The listing builds one solid part. Answer for the finished solid, in the listing's coordinates (mm). Face numbers are marked on the shaded views. A direction names the side the tool comes from. Round coordinates to 2 decimals unless told otherwise and drop trailing zeros. Order: outer loops, then holes, each group sorted by start corner. A loop starts at its lowest first (then second) coordinate and runs counter-clockwise, first axis right, second up. Notation, with made-up numbers: (59, -26.5) -> (107, -26.5) arc R28 ccw to (107, 2.5) -> close; hole circle Ø4 at (-32.5, -14). An arc over 180 degrees is marked (long way). Return JSON: item names as keys, results as strings. Group by question number.
(1) The part is cut by section C-C (z = -7.5). Determine the outline of the cut face in (x, y).
(2) Consider line 1 (Y direction, x = 4.3, z = 0); line 2 (X direction, y = 3.75, z = -0.5); line 3 (X direction, y = 10.25, z = 0.75) (3 decimals). Determine where each line is inside the solid, lowest interval first. Write a range as [from, to].
(3) Each of these flat-tipped pins is pushed along its axis until it touches: pin 1 (0.7 mm diameter, centred on x = 4.5, z = 0, fed in from +Y); pin 2 (1.2 mm diameter, centred on x = 4.5, y = 3.5, fed in from -Z); pin 3 (0.8 mm diameter, centred on y = 10.5, z = 3.5, fed in from +X). Where does it stop, or does it pass through?
(4) Which of the six approach directions +Z, -Z, +X, -X, +Y, -Y give full straight-line access (tool end or side, diameter ignored) to the marked faces 1, 2 and 3?
(5) The part is cut by section B-B (x = 0). Determine the outline of the cut face in (y, z), plus the area to 3 significant figures.
(6) The part is cut by section A-A (z = 0). Determine the outline of the cut face in (x, y) (3 decimals), plus the area to 3 significant figures.
(7) The part is cut by section D-D (y = 5). Determine the outline of the cut face in (x, z), plus the area to 3 significant figures.
(8) Determine the mould class of the marked faces 4, 5 and 6 for opening direction Z: +Z half, -Z half, draft (parallel to the pull), parting line (faces both ways), or undercut.
from build123d import *

# Parameters (mm, degrees)
BOSS_EXTRUDE1_DEPTH       = 2.3
BOSS_EXTRUDE2_START       = 1
BOSS_EXTRUDE2_DEPTH       = 1
SKETCH19_W                = 2
SKETCH19_H                = 1.95
SKETCH19_R                = 0.45
SKETCH19_W_2              = 1.95
SKETCH19_H_2              = 2
CMOS_MOUNTING_HOLES_DEPTH = 3.3
FILLET1_R                 = 0.5
SKETCH21_W                = 7.2
SKETCH21_H                = 7.2
SKETCH21_W_2              = 6
SKETCH21_H_2              = 6
COLUMN_DEPTH              = 6.52
SKETCH22_W                = 6
SKETCH22_H                = 6
COLUMN_EXTRUDED_CUT_DEPTH = 14.675174588
COLUMN_OUTSIDE_FILLET_R   = 1.5
COLUMN_INSIDE_FILLET_R    = 1
SKETCH25_W                = 2.5
SKETCH25_H                = 2.5
SET_SCREW_EXTRUSION_DEPTH = 1.5
SET_SCREW_HOLE_REACH      = 21.834
SKETCH26_R                = 0.55
LARGE_START               = -3.3
SKETCH29_R                = 0.875
LARGE_WIRE_HOLE_DEPTH     = 3.3
FILLET3_R                 = 0.5


with BuildPart() as part:
    # Sketch4 → Boss-Extrude1 (new body)
    with BuildSketch(Plane(origin=(0, 9.37, 0), x_dir=(1, 0, 0), z_dir=(0, 1, 0))):
        with BuildLine():
            Line((-6.55, 5.65), (-6.55, -5.65))
            ThreePointArc((-6.55, -5.65), (-6.286396103, -6.286396103), (-5.65, -6.55))
            Line((-5.65, -6.55), (5.65, -6.55))
            ThreePointArc((5.65, -6.55), (6.286396103, -6.286396103), (6.55, -5.65))
            Line((6.55, -5.65), (6.55, 5.65))
            ThreePointArc((6.55, 5.65), (6.286396103, 6.286396103), (5.65, 6.55))
            Line((5.65, 6.55), (-5.65, 6.55))
            ThreePointArc((-5.65, 6.55), (-6.286396103, 6.286396103), (-6.55, 5.65))
        make_face()
        with BuildLine():
            Line((-5.65, 5.95), (5.65, 5.95))
            ThreePointArc((5.65, 5.95), (5.862132034, 5.862132034), (5.95, 5.65))
            Line((5.95, 5.65), (5.95, -5.65))
            ThreePointArc((5.95, -5.65), (5.862132034, -5.862132034), (5.65, -5.95))
            Line((5.65, -5.95), (-5.65, -5.95))
            ThreePointArc((-5.65, -5.95), (-5.862132034, -5.862132034), (-5.95, -5.65))
            Line((-5.95, -5.65), (-5.95, 5.65))
            ThreePointArc((-5.95, 5.65), (-5.862132034, 5.862132034), (-5.65, 5.95))
        make_face(mode=Mode.SUBTRACT)
    extrude(amount=BOSS_EXTRUDE1_DEPTH)

    # Sketch20 → Boss-Extrude2 (add)
    with BuildSketch(Plane.XZ.offset(-9.37).offset(BOSS_EXTRUDE2_START)):
        with BuildLine():
            Line((5.65, -6.55), (-5.65, -6.55))
            ThreePointArc((-5.65, -6.55), (-6.286396103, -6.286396103), (-6.55, -5.65))
            Line((-6.55, -5.65), (-6.55, 5.65))
            ThreePointArc((-6.55, 5.65), (-6.286396103, 6.286396103), (-5.65, 6.55))
            Line((-5.65, 6.55), (5.65, 6.55))
            ThreePointArc((5.65, 6.55), (6.286396103, 6.286396103), (6.55, 5.65))
            Line((6.55, 5.65), (6.55, -5.65))
            ThreePointArc((6.55, -5.65), (6.286396103, -6.286396103), (5.65, -6.55))
        make_face()
    extrude(amount=-BOSS_EXTRUDE2_DEPTH)

    # Sketch19 → CMOS Mounting Holes (add)
    # profile 1 of 3: a face of its own
    with BuildSketch(Plane(origin=(0, 11.67, 0), x_dir=(1, 0, 0), z_dir=(0, 1, 0))):
        with Locations((0, 7.525)):
            Rectangle(SKETCH19_W, SKETCH19_H)
        with Locations(Location((0, 7.5, 0), (0, 0, 270))):
            Circle(SKETCH19_R, mode=Mode.SUBTRACT)
    # profile 2 of 3: a face of its own
    with BuildSketch(Plane(origin=(0, 11.67, 0), x_dir=(1, 0, 0), z_dir=(0, 1, 0))):
        with Locations((-7.525, -3.5)):
            Rectangle(SKETCH19_W_2, SKETCH19_H_2)
        with Locations(Location((-7.5, -3.5, 0), (0, 0, 270))):
            Circle(SKETCH19_R, mode=Mode.SUBTRACT)
    # profile 3 of 3: a face of its own
    with BuildSketch(Plane(origin=(0, 11.67, 0), x_dir=(1, 0, 0), z_dir=(0, 1, 0))):
        with Locations((7.525, -3.5)):
            Rectangle(SKETCH19_W_2, SKETCH19_H_2)
        with Locations(Location((7.5, -3.5, 0), (0, 0, 270))):
            Circle(SKETCH19_R, mode=Mode.SUBTRACT)
    extrude(amount=-CMOS_MOUNTING_HOLES_DEPTH)

    # Fillet1
    fillet1_edges = [part.edges().sort_by_distance(p)[0] for p in [
        (1, 10.02, -6.55),
        (-1, 10.02, -6.55),
        (-1, 10.02, -8.5),
        (1, 10.02, -8.5),
        (-6.55, 10.02, 2.5),
        (-6.55, 10.02, 4.5),
        (-8.5, 10.02, 4.5),
        (-8.5, 10.02, 2.5),
        (6.55, 10.02, 4.5),
        (6.55, 10.02, 2.5),
        (8.5, 10.02, 2.5),
        (8.5, 10.02, 4.5),
    ]]
    fillet(fillet1_edges, radius=FILLET1_R)

    # Sketch21 → Column (add)
    with BuildSketch(Plane.XZ.offset(-8.37)):
        Rectangle(SKETCH21_W, SKETCH21_H)
        Rectangle(SKETCH21_W_2, SKETCH21_H_2, mode=Mode.SUBTRACT)
    extrude(amount=COLUMN_DEPTH)

    # Sketch22 → Column Extruded Cut (cut, through all)
    with BuildSketch(Plane.XZ.offset(-8.37)):
        Rectangle(SKETCH22_W, SKETCH22_H)
    extrude(amount=-COLUMN_EXTRUDED_CUT_DEPTH, mode=Mode.SUBTRACT)

    # Column Outside Fillet
    column_outside_fillet_edges = [part.edges().sort_by_distance(p)[0] for p in [
        (-3.6, 5.11, 3.6),
        (-3.6, 5.11, -3.6),
        (3.6, 5.11, -3.6),
        (3.6, 5.11, 3.6),
    ]]
    fillet(column_outside_fillet_edges, radius=COLUMN_OUTSIDE_FILLET_R)

    # Column Inside Fillet
    column_inside_fillet_edges = [part.edges().sort_by_distance(p)[0] for p in [
        (-3, 5.61, -3),
        (3, 5.61, -3),
        (3, 5.61, 3),
        (-3, 5.61, 3),
    ]]
    fillet(column_inside_fillet_edges, radius=COLUMN_INSIDE_FILLET_R)

    # Sketch25 → Set Screw Extrusion (add)
    with BuildSketch(Plane(origin=(3.6, 0, 0), x_dir=(0, 0, -1), z_dir=(1, 0, 0))):
        with Locations((0, 3.1)):
            Rectangle(SKETCH25_W, SKETCH25_H)
    extrude(amount=SET_SCREW_EXTRUSION_DEPTH)

    # Sketch26 → Set Screw Hole (cut, up to next)
    with BuildSketch(Plane(origin=(5.1, 0, 0), x_dir=(0, 0, -1), z_dir=(1, 0, 0)), mode=Mode.PRIVATE) as set_screw_hole_sk1:
        with Locations((0, 3.1)):
            Circle(SKETCH26_R)
    set_screw_hole_tool1 = extrude(set_screw_hole_sk1.sketch, amount=-SET_SCREW_HOLE_REACH, mode=Mode.PRIVATE) & part.part
    add(set_screw_hole_tool1.solids().sort_by_distance((5.1, 3.1, 0))[0], mode=Mode.SUBTRACT)

    # Sketch29 → Large Wire Hole (add)
    with BuildSketch(Plane(origin=(0, 11.67, 0), x_dir=(1, 0, 0), z_dir=(0, 1, 0)).offset(LARGE_START)):
        with BuildLine():
            Line((6.55, -2), (6.55, 1.375))
            Line((6.55, 1.375), (8.925, 1.375))
            Line((8.925, 1.375), (8.925, -1.375))
            Line((8.925, -1.375), (8.5, -3))
            ThreePointArc((8.5, -3), (8.353553391, -2.646446609), (8, -2.5))
            Line((8, -2.5), (7.05, -2.5))
            ThreePointArc((7.05, -2.5), (6.696446609, -2.353553391), (6.55, -2))
        make_face()
        with Locations(Location((7.55, 0, 0), (0, 0, 270))):
            Circle(SKETCH29_R, mode=Mode.SUBTRACT)
    extrude(amount=LARGE_WIRE_HOLE_DEPTH)

    # Fillet3
    fillet3_edges = [part.edges().sort_by_distance(p)[0] for p in [
        (6.55, 10.02, -1.375),
        (8.925, 10.02, -1.375),
    ]]
    fillet(fillet3_edges, radius=FILLET3_R)


solid = part.part
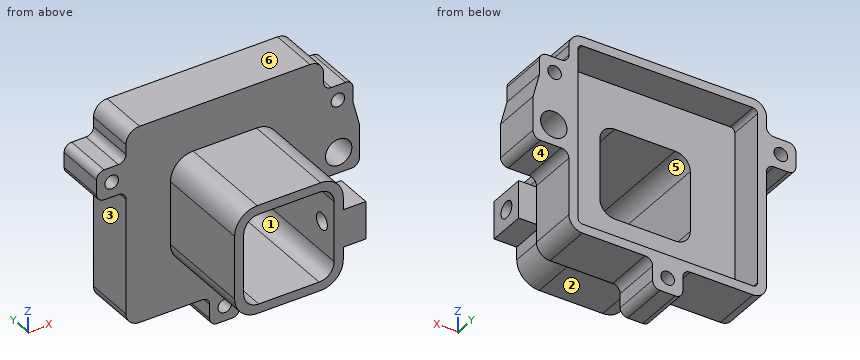
Answer below:
{
 "1": {"outline": "(-1, 8.37) -> (-0.45, 8.37) -> (-0.45, 11.67) -> (-1, 11.67) -> close; (0.45, 8.37) -> (1, 8.37) -> (1, 11.67) -> (0.45, 11.67) -> close"},
 "2": {"line 1": "y = [1.85, 2.55], [3.65, 4.35], [8.37, 9.37]", "line 2": "x = [-3.6, -3], [3, 5.1]", "line 3": "x = [-6.55, -5.95], [5.95, 7.099], [8.001, 8.925]"},
 "3": {"pin 1": "stops at y = 9.37", "pin 2": "stops at z = -1.25", "pin 3": "stops at x = 8.5"},
 "4": {"face 1": "+Y, -Y", "face 2": "-Z, +X, -X, -Y", "face 3": "-Z, -X, +Y, -Y"},
 "5": {"outline": "(1.85, -3.6) -> (8.37, -3.6) -> (8.37, -7.05) -> (11.67, -7.05) -> (11.67, -5.95) -> (9.37, -5.95) -> (9.37, -3) -> (1.85, -3) -> close; (1.85, 3) -> (9.37, 3) -> (9.37, 5.95) -> (11.67, 5.95) -> (11.67, 6.55) -> (8.37, 6.55) -> (8.37, 3.6) -> (1.85, 3.6) -> close; (8.37, -8.5) -> (11.67, -8.5) -> (11.67, -7.95) -> (8.37, -7.95) -> close", "area": "21.1 mm²"},
 "6": {"outline": "(-6.55, 8.37) -> (-3.6, 8.37) -> (-3.6, 1.85) -> (-3, 1.85) -> (-3, 9.37) -> (-5.95, 9.37) -> (-5.95, 11.67) -> (-6.55, 11.67) -> close; (3, 1.85) -> (5.1, 1.85) -> (5.1, 2.55) -> (3, 2.55) -> close; (3, 3.65) -> (5.1, 3.65) -> (5.1, 4.35) -> (3.6, 4.35) -> (3.6, 8.37) -> (6.675, 8.37) -> (6.675, 11.67) -> (5.95, 11.67) -> (5.95, 9.37) -> (3, 9.37) -> close; (8.425, 8.37) -> (8.925, 8.37) -> (8.925, 11.67) -> (8.425, 11.67) -> close", "area": "21.2 mm²"},
 "7": {"outline": "(-3.6, -2.1) arc R1.5 ccw to (-2.1, -3.6) -> (2.1, -3.6) arc R1.5 ccw to (3.6, -2.1) -> (3.6, 2.1) arc R1.5 ccw to (2.1, 3.6) -> (-2.1, 3.6) arc R1.5 ccw to (-3.6, 2.1) -> close; hole (-3, -2) arc R1 ccw to (-2, -3) -> (2, -3) arc R1 ccw to (3, -2) -> (3, 2) arc R1 ccw to (2, 3) -> (-2, 3) arc R1 ccw to (-3, 2) -> close", "area": "14.8 mm²"},
 "8": {"face 4": "-Z half", "face 5": "undercut", "face 6": "+Z half"}
}
